Design review of the part shown in the three views and the two pictorial views. Dimensions are in mm from the part's minimum x, y and z. A direction names the side the tool comes from. Give positions to 0.01 mm unless a question says otherwise; leave off trailing zeros. Loops run counter-clockwise (first coordinate to the right, second up) from the corner with the lowest first, then second, coordinate; pieces in that order, holes last. Notation, with made-up numbers: (0, -15) - (18, -15) arc R24 cw to (18, 11) - close; hole circle Ø11 at (-17.5, 34.25). An arc over 180 degrees is marked (long way). Answer in a Markdown table with one row per item.
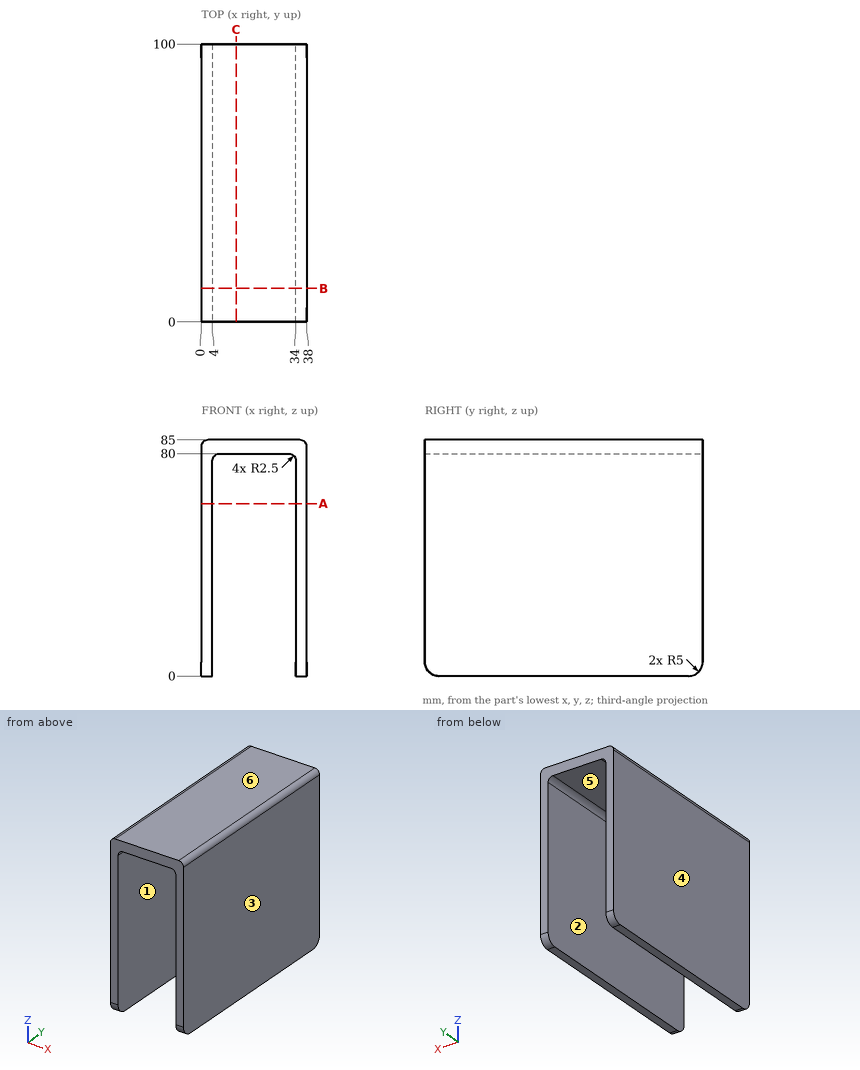
1. Mouldability with a two-part tool opening along X and no side actions: class the marked faces 1, 2, 3 and 4 as released by +X, released by -X, zero draft, split by the parting line, or undercut.
Values:
| item | result |
|---|---|
| face 1 | undercut |
| face 2 | undercut |
| face 3 | released by +X |
| face 4 | released by -X |
2. We need section A-A, the plane z = 62. Give the boundary of the cut face in (x, y), and give its area (3 significant figures).
Values:
| item | result |
|---|---|
| outline | (0, 0) - (4, 0) - (4, 100) - (0, 100) - close; (34, 0) - (38, 0) - (38, 100) - (34, 100) - close |
| area | 800 mm^2 |
3. We need section B-B, the plane y = 12. Give the boundary of the cut face in (x, z), and give its area (3 significant figures).
Values:
| item | result |
|---|---|
| outline | (0, 0) - (4, 0) - (4, 77.5) arc R2.5 cw to (6.5, 80) - (31.5, 80) arc R2.5 cw to (34, 77.5) - (34, 0) - (38, 0) - (38, 82.5) arc R2.5 ccw to (35.5, 85) - (2.5, 85) arc R2.5 ccw to (0, 82.5) - close |
| area | 830 mm^2 |
4. Clearance check with a flat-ended pin moving along its axis: pin 1 (20 mm diameter, centred on x = 21, y = 59.5, fed in from -Z). State where the tip first meets the part, or that it passes through.
Values:
| item | result |
|---|---|
| pin 1 | stops at z = 80 |
5. For the marked faces 5 and 6, list the 3-axis set-ups (+Z, -Z, +X, -X, +Y, -Y) from which the entire face can be reached by the end or side of a thin tool; tool diameter is ignored.
Values:
| item | result |
|---|---|
| face 5 | -Z, +Y, -Y |
| face 6 | +Z, +X, -X, +Y, -Y |
6. We need section C-C, the plane x = 12.5. Give the boundary of the cut face in (y, z), and give its area (3 significant figures).
Values:
| item | result |
|---|---|
| outline | (0, 80) - (100, 80) - (100, 85) - (0, 85) - close |
| area | 500 mm^2 |
7. Wall thickness on line 1 (X direction, y = 27.5, z = 20); line 2 (Z direction, x = 26.5, y = 88); line 3 (Z direction, x = 32.5, y = 16.5): over which ranges is each line inside the solid? List them lowest first. Write a range as [from, to].
Values:
| item | result |
|---|---|
| line 1 | x = [0, 4], [34, 38] |
| line 2 | z = [80, 85] |
| line 3 | z = [79.79, 85] |
